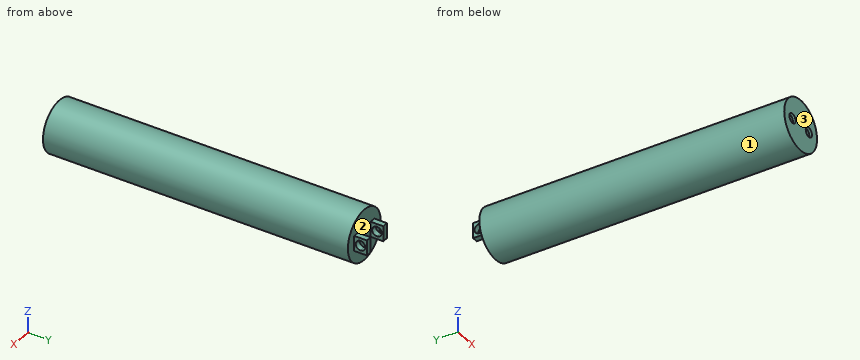
```python
from build123d import *

# Parameters (mm, degrees)
SKETCH1_R           = 25.4
BOSS_EXTRUDE1_DEPTH = 304.8
SKETCH3_W           = 5.753643288
SKETCH3_H           = 15.213425176
SKETCH3_W_2         = 5.733174908
BOSS_EXTRUDE2_DEPTH = 12.7
CUT_EXTRUDE2_DEPTH  = 62.738
SKETCH6_R           = 4.7625
CUT_EXTRUDE3_DEPTH  = 2.54


with BuildPart() as part:
    # Sketch1 → Boss-Extrude1 (new body)
    with BuildSketch(Plane(origin=(0, 0, 0), x_dir=(1, 0, 0), z_dir=(0, 1, 0))):
        with Locations(Location((0, 0, 0), (0, 0, 90))):
            Circle(SKETCH1_R)
    extrude(amount=BOSS_EXTRUDE1_DEPTH)

    # Sketch3 → Boss-Extrude2 (add)
    with BuildSketch(Plane(origin=(0, 304.8, 0), x_dir=(1, 0, 0), z_dir=(0, 1, 0))):
        with Locations((12.7, 0)):
            Rectangle(SKETCH3_W, SKETCH3_H)
        with Locations((-12.7, 0)):
            Rectangle(SKETCH3_W_2, SKETCH3_H)
    extrude(amount=BOSS_EXTRUDE2_DEPTH)

    # Sketch4 → Cut-Extrude2 (cut)
    with BuildSketch(Plane(origin=(15.576821644, 0, 0), x_dir=(0, 0, -1), z_dir=(1, 0, 0))):
        with BuildLine():
            ThreePointArc((4.826, 311.15), (3.412497326, 314.562497326), (0, 315.976))
            Line((0, 315.976), (0, 306.324))
            ThreePointArc((0, 306.324), (3.412497326, 307.737502674), (4.826, 311.15))
        make_face()
        with BuildLine():
            Line((0, 306.324), (0, 315.976))
            ThreePointArc((0, 315.976), (-4.826, 311.15), (0, 306.324))
        make_face()
    extrude(amount=-CUT_EXTRUDE2_DEPTH, mode=Mode.SUBTRACT)

    # Sketch6 → Cut-Extrude3 (cut)
    with BuildSketch(Plane.XZ):
        with Locations(Location((-12.7, 0, 0), (0, 0, 270))):
            Circle(SKETCH6_R)
        with Locations(Location((12.7, 0, 0), (0, 0, 270))):
            Circle(SKETCH6_R)
    extrude(amount=-CUT_EXTRUDE3_DEPTH, mode=Mode.SUBTRACT)


solid = part.part
```
Check sheet for the modelled part. Datum: model origin and axes. Units: mm. Face numbers are marked on the shaded views. Round coordinates to 2 decimals unless told otherwise and drop trailing zeros. Loops run counter-clockwise (first coordinate to the right, second up) from the corner with the lowest first, then second, coordinate; pieces in that order, holes last. Notation, with made-up numbers: M 26.5,36 L 33.5,36 A18 cw 33.5,50 Z; hole C 84.25,3 d5. An arc over 180 degrees is marked long. Answer as a JSON object with one key per item and string values.
1. Section check C-C (x = 0). Record the boundary of the cut face in (y, z).
Reply:
{"outline": "M 0,-25.4 L 304.8,-25.4 L 304.8,25.4 L 0,25.4 Z"}
2. Scan lines: line 1 (X direction, y = 1.15, z = 0); line 2 (Y direction, x = 9, z = 0); line 3 (Y direction, x = 0, z = 15). Record each from-to range of solid material in increasing order.
Reply:
{"line 1": "x = -25.4 to -17.46, -7.94 to 7.94, 17.46 to 25.4", "line 2": "y = 2.54 to 304.8", "line 3": "y = 0 to 304.8"}
3. Section check D-D (z = -18.5). Record the boundary of the cut face in (x, y), plus the area to 3 significant figures.
Reply:
{"outline": "M -17.4,0 L 17.4,0 L 17.4,304.8 L -17.4,304.8 Z", "area": "10,600 mm²"}
4. Mould release check, pull along X, two halves, no side actions. Record for the marked faces 1, 2 and 3: pulls with the +X half, pulls with the -X half, needs draft (parallel to the pull), parting line crosses it, or undercut.
Reply:
{"face 1": "parting line crosses it", "face 2": "undercut", "face 3": "needs draft"}
5. Section check A-A (x = -12.7). Record the boundary of the cut face in (y, z), plus the area to 3 significant figures.
Reply:
{"outline": "M 0,-22 L 304.8,-22 L 304.8,-7.61 L 317.5,-7.61 L 317.5,7.61 L 304.8,7.61 L 304.8,22 L 0,22 L 0,4.76 L 2.54,4.76 L 2.54,-4.76 L 0,-4.76 Z; hole C 311.15,0 d9.65", "area": "13,500 mm²"}
6. Gauge pin test, flat ends, axial feed: P1, Ø6.5, axis at x = -13, y = 314, coming from the +Z side; P2, Ø6.5, axis at x = 12, y = 314, coming from the -Z side; P3, Ø3, axis at x = -17.5, z = 7.5, coming from the -Y side; P4, Ø3, axis at x = -12.5, z = 2.5, coming from the -Y side. Record the tip position at first contact, or that the pin passes through.
Reply:
{"P1": "stops at z = 7.61", "P2": "stops at z = -7.61", "P3": "stops at y = 0", "P4": "stops at y = 2.54"}
7. Section check B-B (y = 178.5). Record the boundary of the cut face in (x, z).
Reply:
{"outline": "C 0,0 d50.8"}
